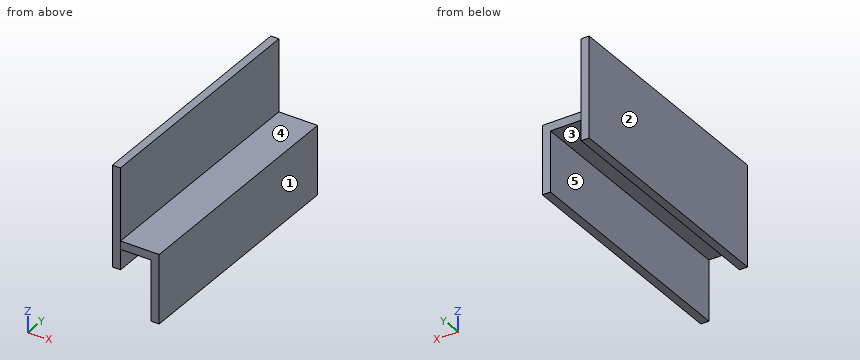
```python
from build123d import *

# Parameters (mm, degrees)
F0_W     = 152.4
F0_H     = 63.5
F1_DEPTH = 5.08
F3_W     = 152.400844
F3_H     = 5.193346
F4_DEPTH = 24.384
F5_W     = 5.08
F5_H     = 152.400844
F6_DEPTH = 38.1


with BuildPart() as f1:
    # F0 (on Right) → F1 (new body)
    with BuildSketch(Plane.YZ):
        Rectangle(F0_W, F0_H)
    extrude(amount=-F1_DEPTH)

    # F3 (on face) → F4 (join)
    with BuildSketch(Plane.YZ):
        with Locations((0.000302, -16.370494)):
            Rectangle(F3_W, F3_H)
    extrude(amount=F4_DEPTH)

    # F5 (on face) → F6 (join)
    with BuildSketch(Plane(origin=(0, 0, -18.967167), x_dir=(1, 0, 0), z_dir=(0, 0, -1))):
        with Locations((21.844, -0.000302)):
            Rectangle(F5_W, F5_H)
    extrude(amount=F6_DEPTH)


solid = f1.part
```
Here's how the part is built. I have some questions about the finished solid (model axes, mm). Face numbers are marked on the shaded views. A direction names the side the tool comes from. Round coordinates to 2 decimals unless told otherwise and drop trailing zeros. Order: outer loops, then holes, each group sorted by start corner. A loop starts at its lowest first (then second) coordinate and runs counter-clockwise, first axis right, second up. Notation, with made-up numbers: (74, 33.5) -> (102, 33.5) arc R21 ccw to (102, 63.5) -> close; hole circle Ø10 at (9, 2). An arc over 180 degrees is marked (long way). Use a Markdown table: item, result. Add a question column.
(1) For the marked faces 4 and 5, which set-ups out of +Z, -Z, +X, -X, +Y, -Y let a thin tool reach every point of the face, with its end or its side?
(2) Suppose I cut it at A-A, the plane y = -8. Please give me the cut outline in (x, z).
(3) I need wall thicknesses on line 1 along X through (y, z) = (-25, -25.5); line 2 along Z through (x, y) = (4.75, -39); line 3 along Z through (x, y) = (-2.5, -12). Which ranges of each line are inside material? Lowest first, please.
(4) If we mould it in two halves opening along X, with no side actions, what happens to the marked faces 1, 2 and 3? For each: released by +X, released by -X, zero draft, split by the parting line, or undercut.
(5) Suppose I cut it at C-C, the plane z = -37. Please give me the cut outline in (x, y).
(6) For pin 1 Ø4 at (x, y) = (-2.5, -23.5) entering from -Z; pin 2 Ø13.5 at (y, z) = (19, 9.5) entering from +X; pin 3 Ø12 at (x, y) = (7, -29) entering from -Z, each with a flat end and sliding along its axis, tell me the tip position at first contact or that it passes through.
(7) Suppose I cut it at B-B, the plane x = 5. Please give me the cut outline in (y, z), and give its area (3 significant figures).
Verdict:
| question | item | result |
|---|---|---|
| 1 | face 4 | +Z, +X, +Y, -Y |
| 1 | face 5 | -Z, +Y, -Y |
| 2 | outline | (-5.08, -31.75) -> (0, -31.75) -> (0, -18.97) -> (19.3, -18.97) -> (19.3, -57.07) -> (24.38, -57.07) -> (24.38, -13.77) -> (0, -13.77) -> (0, 31.75) -> (-5.08, 31.75) -> close |
| 3 | line 1 | -5.08 to 0, 19.3 to 24.38 |
| 3 | line 2 | -18.97 to -13.77 |
| 3 | line 3 | -31.75 to 31.75 |
| 4 | face 1 | released by +X |
| 4 | face 2 | released by -X |
| 4 | face 3 | undercut |
| 5 | outline | (19.3, -76.2) -> (24.38, -76.2) -> (24.38, 76.2) -> (19.3, 76.2) -> close |
| 6 | pin 1 | z = -31.75 |
| 6 | pin 2 | x = 0 |
| 6 | pin 3 | z = -18.97 |
| 7 | outline | (-76.2, -18.97) -> (76.2, -18.97) -> (76.2, -13.77) -> (-76.2, -13.77) -> close |
| 7 | area | 791 mm2 |
